Autodesk Inventor part; units mm, degrees
ref_plane "YZ Plane" through (0, 0, 0) normal (1, 0, 0) x (0, 1, 0)
ref_plane "XZ Plane" through (0, 0, 0) normal (0, 1, 0) x (-1, 0, 0)
ref_plane "XY Plane" through (0, 0, 0) normal (0, 0, 1) x (1, 0, 0)
sketch "Sketch1" plane through (0, 0, 0) normal (0, 1, 0) x (-1, 0, 0)
  line L0 (-152.4, 234.95) -> (152.4, 234.95)
  line L1 (152.4, 234.95) -> (152.4, -234.95)
  line L2 (152.4, -234.95) -> (-152.4, -234.95)
  line L3 (-152.4, -234.95) -> (-152.4, 234.95)
  line L4 (-152.4, 234.95) -> (152.4, -234.95) construction
  line L5 (152.4, 234.95) -> (-152.4, -234.95) construction
  circle A0 centre (127, -79.375) radius 25.4 construction
  circle A1 centre (127, 79.375) radius 25.4 construction
  circle A2 centre (7.5484, 152.4) radius 25.4 construction
  circle A3 centre (7.5484, -152.4) radius 25.4 construction
  circle A4 centre (-122.9151, -203.2) radius 25.4 construction
  circle A5 centre (-122.9151, 203.2) radius 25.4 construction
  point P0 (0, 0)
  dimension "d0" = 304.8
  dimension "d1" = 469.9
  dimension "d2" = 158.75
  dimension "d3" = 50.8
  dimension "d4" = 50.8
  dimension "d5" = 79.375
  dimension "d6" = 50.8
  dimension "d7" = 50.8
  dimension "d8" = 50.8
  dimension "d9" = 50.8
  dimension "d10" = 406.4
  dimension "d11" = 304.8
  dimension "d12" = 152.4
  dimension "d14" = 203.2
  dimension "d17" = 140.0048
  dimension "d18" = 140.0048
  dimension "d19" = 25.4
extrude "Extrusion1" add sketch "Sketch1" along normal blind 6.35
hole "Hole1" at (-127, 0, 79.375) at (-127, 0, -79.375) at (-7.5484, 0, 152.4) at (122.9151, 0, 203.2) at (-7.5484, 0, -152.4) at (122.9151, 0, -203.2) direction (0, 1, 0) diameter 28.575 end through all
equation "\"d3\" = d4"
equation "\"d6\" = d4"
equation "\"d7\" = d4"
equation "\"d8\" = d4"
equation "\"d9\" = d4"
properties part number "Int1-001" material "Aluminum 6061"
Read the model definition and answer for the solid it produces. Units are mm, in the model's axes. Round coordinates to 2 decimals unless told otherwise and drop trailing zeros. Loops run counter-clockwise (first coordinate to the right, second up) from the corner with the lowest first, then second, coordinate; pieces in that order, holes last. Notation, with made-up numbers: (1.5, 12) -> (40.5, 12) arc R10 ccw to (40.5, 27) -> close; hole circle Ø10 at (23, -14). An arc over 180 degrees is marked (long way). One line per item, written item: value.
1) A cutting plane is placed at D-D (z = -147). Determine the outline of the cut face in (x, y).
Answer list:
outline: (-152.4, 0) -> (-20.78, 0) -> (-20.78, 6.35) -> (-152.4, 6.35) -> close; (5.68, 0) -> (152.4, 0) -> (152.4, 6.35) -> (5.68, 6.35) -> close
2) A cutting plane is placed at A-A (x = -127). Determine the outline of the cut face in (y, z), and give its area (3 significant figures).
Answer list:
outline: (0, -234.95) -> (6.35, -234.95) -> (6.35, -93.66) -> (0, -93.66) -> close; (0, -65.09) -> (6.35, -65.09) -> (6.35, 65.09) -> (0, 65.09) -> close; (0, 93.66) -> (6.35, 93.66) -> (6.35, 234.95) -> (0, 234.95) -> close
area: 2,620 mm²
3) A cutting plane is placed at C-C (y = 1.5). Give the number of separate pieces and of enclosed holes in the cut face, and give its area (3 significant figures).
Answer list:
separate pieces: 1
enclosed holes: 6
area: 139,000 mm²
4) A cutting plane is placed at B-B (z = 203.2). Determine the outline of the cut face in (x, y), and give its area (3 significant figures).
Answer list:
outline: (-152.4, 0) -> (108.63, 0) -> (108.63, 6.35) -> (-152.4, 6.35) -> close; (137.2, 0) -> (152.4, 0) -> (152.4, 6.35) -> (137.2, 6.35) -> close
area: 1,750 mm²
5) Consider L1, parallel to Z at x = -127, y = 2.5; L2, parallel to Z at x = -8.5, y = 5.75; L3, parallel to X at y = 3.75, z = -152.4. Determine where each line is inside the solid, lowest interval first. Write a range as [from, to].
Answer list:
L1: z = [-234.95, -93.66], [-65.09, 65.09], [93.66, 234.95]
L2: z = [-234.95, -166.66], [-138.14, 138.14], [166.66, 234.95]
L3: x = [-152.4, -21.84], [6.74, 152.4]
6) The mould has two halves that part along Z. Classify faces 1 (the face through (128.387, 3.219, -216.398)), 2 (the face through (2, 0, 3)): pulls with the +Z half, pulls with the -Z half, needs draft (parallel to the pull), parting line crosses it, or undercut.
Answer list:
face 1: undercut
face 2: needs draft
